```python
from build123d import *

# Parameters (mm, degrees)
SKETCH1_R           = 7
BOSS_EXTRUDE1_DEPTH = 5
SKETCH2_R           = 4
CUT_EXTRUDE1_DEPTH  = 6


with BuildPart() as part:
    # Sketch1 → Boss-Extrude1 (new body)
    with BuildSketch(Plane(origin=(0, 0, 0), x_dir=(1, 0, 0), z_dir=(0, 1, 0))):
        with BuildLine():
            Line((-449.708642176, 415.631578947), (-361.296475424, 415.631578947))
            Line((-361.296475424, 415.631578947), (-361.296475424, 215.631578947))
            Line((-361.296475424, 215.631578947), (-449.708642176, 215.631578947))
            Line((-449.708642176, 215.631578947), (-449.708642176, 105.631578947))
            ThreePointArc((-449.708642176, 105.631578947), (-452.637574364, 98.560511136), (-459.708642176, 95.631578947))
            Line((-459.708642176, 95.631578947), (-499.708642176, 95.631578947))
            ThreePointArc((-499.708642176, 95.631578947), (-506.779709988, 98.560511136), (-509.708642176, 105.631578947))
            Line((-509.708642176, 105.631578947), (-509.708642176, 215.631578947))
            Line((-509.708642176, 215.631578947), (-701.296475424, 215.631578947))
            Line((-701.296475424, 215.631578947), (-701.296475424, 415.631578947))
            Line((-701.296475424, 415.631578947), (-509.708642176, 415.631578947))
            Line((-509.708642176, 415.631578947), (-509.708642176, 525.631578947))
            ThreePointArc((-509.708642176, 525.631578947), (-506.779709988, 532.702646759), (-499.708642176, 535.631578947))
            Line((-499.708642176, 535.631578947), (-459.708642176, 535.631578947))
            ThreePointArc((-459.708642176, 535.631578947), (-452.637574364, 532.702646759), (-449.708642176, 525.631578947))
            Line((-449.708642176, 525.631578947), (-449.708642176, 415.631578947))
        make_face()
        with Locations((-479.708642176, 475.631578947)):
            Circle(SKETCH1_R, mode=Mode.SUBTRACT)
        with Locations((-479.708642176, 155.631578947)):
            Circle(SKETCH1_R, mode=Mode.SUBTRACT)
    extrude(amount=BOSS_EXTRUDE1_DEPTH)

    # Sketch2 → Cut-Extrude1 (cut, through all)
    with BuildSketch(Plane(origin=(0, 5, 0), x_dir=(1, 0, 0), z_dir=(0, 1, 0))):
        with Locations((-479.708642176, 195.631578947)):
            Circle(SKETCH2_R)
        with Locations((-479.708642176, 115.631578947)):
            Circle(SKETCH2_R)
        with Locations((-479.708642176, 515.631578947)):
            Circle(SKETCH2_R)
        with Locations((-479.708642176, 435.631578947)):
            Circle(SKETCH2_R)
    extrude(amount=-CUT_EXTRUDE1_DEPTH, mode=Mode.SUBTRACT)


solid = part.part
```
The model under review builds one solid part; all positions refer to its coordinate system, in mm. Round coordinates to 2 decimals unless told otherwise and drop trailing zeros. Loops run counter-clockwise (first coordinate to the right, second up) from the corner with the lowest first, then second, coordinate; pieces in that order, holes last. Notation, with made-up numbers: M -32,56 L 13,56 A33 cw 13,84 Z; hole C 72.5,35 d4. An arc over 180 degrees is marked long. Answer as a JSON object with one key per item and string values.
(1) Take a section at A-A on y = 0.75. Give the boundary of the cut face in (x, z), and give its area (3 significant figures).
Resolved:
{"outline": "M -701.3,-415.63 L -509.71,-415.63 L -509.71,-525.63 A10 ccw -499.71,-535.63 L -459.71,-535.63 A10 ccw -449.71,-525.63 L -449.71,-415.63 L -361.3,-415.63 L -361.3,-215.63 L -449.71,-215.63 L -449.71,-105.63 A10 ccw -459.71,-95.63 L -499.71,-95.63 A10 ccw -509.71,-105.63 L -509.71,-215.63 L -701.3,-215.63 Z; hole C -479.71,-475.63 d14; hole C -479.71,-155.63 d14; hole C -479.71,-515.63 d8; hole C -479.71,-435.63 d8; hole C -479.71,-195.63 d8; hole C -479.71,-115.63 d8", "area": "81,800 mm²"}
(2) Draft analysis for pull direction Z (two halves, no side actions). For faces 1 (the flat face through (-529, 5, -319)), 2 (the cylindrical face through (-452.716, 2.465, -532.78)), 3 (the cylindrical face through (-486.7, 2.46, -155.94)), 4 (the cylindrical face through (-481.23, 2.46, -468.8)), state which applies: released by +Z, released by -Z, zero draft, split by the parting line, or undercut.
Resolved:
{"face 1": "zero draft", "face 2": "released by -Z", "face 3": "undercut", "face 4": "undercut"}
(3) Take a section at C-C on x = -432.5. Give the boundary of the cut face in (y, z), and give its area (3 significant figures).
Resolved:
{"outline": "M 0,-415.63 L 5,-415.63 L 5,-215.63 L 0,-215.63 Z", "area": "1,000 mm²"}
(4) To check wall thickness, follow line 1 along Z through (x, y) = (-421.5, 1.9); line 2 along X through (y, z) = (1.3, -475.5); line 3 along X through (y, z) = (3.45, -208.5). State the ranges of each line that lie inside material, in increasing order.
Resolved:
{"line 1": "-415.63 to -215.63", "line 2": "-509.71 to -486.71, -472.71 to -449.71", "line 3": "-509.71 to -449.71"}
(5) Take a section at B-B on z = -178. Give the boundary of the cut face in (x, y).
Resolved:
{"outline": "M -509.71,0 L -449.71,0 L -449.71,5 L -509.71,5 Z"}
(6) Clearance check with flat-ended pins moving along their axes: P1, Ø5, axis at x = -479.71, z = -195.63, coming from the -Y side; P2, Ø1, axis at x = -572, y = 4.5, coming from the +Z side; P3, Ø2.5, axis at y = 2, z = -477.5, coming from the +X side. State where each tip first meets the part, or that it passes through.
Resolved:
{"P1": "through", "P2": "z = -215.63", "P3": "x = -449.71"}
